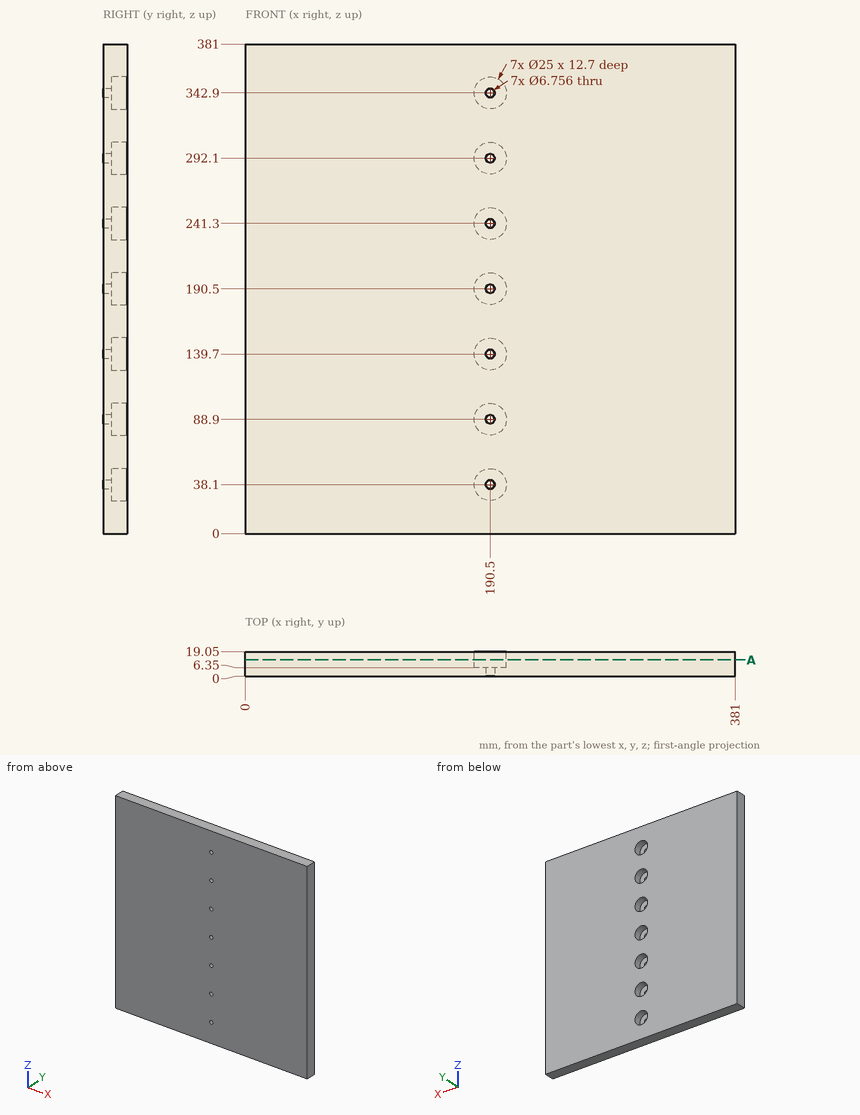
Geometry: see drawing. Coordinates: mm, zero at the bounding-box minimum. Give positions to 0.01 mm unless a question says otherwise; leave off trailing zeros. Loops run counter-clockwise (first coordinate to the right, second up) from the corner with the lowest first, then second, coordinate; pieces in that order, holes last. Notation, with made-up numbers: (-24.5, 2) - (3.5, 2) arc R22 ccw to (3.5, 11) - close; hole circle Ø4 at (-14.75, -17.75). An arc over 180 degrees is marked (long way). Use CSV: the item, a comma, the result in double quotes. Start each with the question number.
Item 1: Contact query for flat-ended pins moving along their axis: P1, Ø15, axis at x = 190.5, z = 38.1, coming from the -Y side; P2, Ø9, axis at x = 190.5, z = 241.3, coming from the +Y side. Output: stop coordinate, or through.
Item 2: Line query: line 1 (X direction, y = 11.75, z = 342.9); line 2 (X direction, y = 2, z = 241.3). Output: solid intervals per line, ascending.
Item 3: Section A-A on y = 12.5. Return loops of the section in (x, z).
Ans:
1,P1,"stops at y = 0"
1,P2,"stops at y = 6.35"
2,line 1,"x = 0 to 178, 203 to 381"
2,line 2,"x = 0 to 187.12, 193.88 to 381"
3,outline,"(0, 0) - (381, 0) - (381, 381) - (0, 381) - close; hole circle Ø25 at (190.5, 38.1); hole circle Ø25 at (190.5, 88.9); hole circle Ø25 at (190.5, 139.7); hole circle Ø25 at (190.5, 190.5); hole circle Ø25 at (190.5, 241.3); hole circle Ø25 at (190.5, 292.1); hole circle Ø25 at (190.5, 342.9)"
